Read the model definition and answer for the solid it produces. Units are mm, in the model's axes. Coordinates: 2 decimals unless noted, no trailing zeros. Loops run counter-clockwise (first coordinate to the right, second up) from the corner with the lowest first, then second, coordinate; pieces in that order, holes last.
from build123d import *

# Parameters (mm, degrees)
F0_W     = 75
F0_H     = 46
F1_DEPTH = 18
F2_R     = 8.99999


# Not quite as in the source:
# - a fillet or chamfer is up to 0.001 mm smaller than in the source, because OpenCascade refuses the exact size


with BuildPart() as f1:
    # F0 (on Top) → F1 (new body)
    with BuildSketch(Plane.XY):
        Rectangle(F0_W, F0_H)
    extrude(amount=F1_DEPTH)

    # F2 (radius 9 in the source; OpenCascade refuses exactly that, so slightly less here)
    f2_edges = [f1.edges().sort_by_distance(p)[0] for p in [
        (37.5, 0, 18),
        (37.5, 0, 0),
        (-37.5, 0, 0),
        (-37.5, 0, 18),
    ]]
    fillet(f2_edges, radius=F2_R)


solid = f1.part
Item 1: Find the intervals of material crossed by line 1 along Z through (x, y) = (29, -13.5); line 2 along X through (y, z) = (5, 2.75); line 3 along X through (y, z) = (-4.5, 7.5), in increasing order.
Numbers:
line 1: z = 0.01 to 17.99
line 2: x = -34.98 to 34.98
line 3: x = -37.37 to 37.37
Item 2: A cutting plane is placed at C-C on x = -32. Determine the outline of the cut face in (y, z).
Numbers:
outline: (-23, 0.71) - (23, 0.71) - (23, 17.29) - (-23, 17.29) - close
Item 3: A cutting plane is placed at B-B on z = 16.25. Determine the outline of the cut face in (x, y).
Numbers:
outline: (-33.83, -23) - (33.83, -23) - (33.83, 23) - (-33.83, 23) - close
